Autodesk Inventor part; units mm, degrees
ref_plane "YZ Plane" through (0, 0, 0) normal (1, 0, 0) x (0, 1, 0)
ref_plane "XZ Plane" through (0, 0, 0) normal (0, 1, 0) x (-1, 0, 0)
ref_plane "XY Plane" through (0, 0, 0) normal (0, 0, 1) x (1, 0, 0)
sketch "Sketch1" plane through (0, 0, 0) normal (0, 1, 0) x (-1, 0, 0)
  line L0 (20.193, 15.748) -> (-20.193, 15.748)
  line L1 (-20.193, -15.748) -> (20.193, -15.748)
  line L2 (20.193, 15.748) -> (-20.193, -15.748) construction
  line L3 (-20.193, 15.748) -> (20.193, -15.748) construction
  line L4 (26.2784, 0) -> (13.1572, 0) construction
  line L5 (26.2784, 4.445) -> (20.193, 4.445)
  line L6 (20.193, -4.445) -> (26.2784, -4.445)
  arc A0 (26.2784, -4.445) -> (26.2784, 4.445) centre (26.2784, 0) ccw
  line L7 (0, -15.748) -> (0, 15.748) construction
  line L8 (-26.2784, 4.445) -> (-20.193, 4.445)
  line L9 (-20.193, -4.445) -> (-26.2784, -4.445)
  arc A1 (-26.2784, 4.445) -> (-26.2784, -4.445) centre (-26.2784, 0) ccw
  line L10 (20.193, -15.748) -> (20.193, -4.445)
  line L11 (20.193, 4.445) -> (20.193, 15.748)
  line L12 (-20.193, 15.748) -> (-20.193, 4.445)
  line L13 (-20.193, -4.445) -> (-20.193, -15.748)
  circle A2 centre (-26.2784, 0) radius 2.5527
  circle A3 centre (26.2784, 0) radius 2.5527
  point P0 (0, 0)
  point P1 (19.7178, 0)
  dimension "d0" = 40.386
  dimension "d1" = 31.496
  dimension "d2" = 8.89
  dimension "d5" = 5.1054
  dimension "d6" = 5.1054
extrude "Extrusion2" add sketch "Sketch1" along normal blind 6.35
sketch "Sketch2" plane through (0, 6.35, 0) normal (0, 1, 0) x (1, 0, 0)
  line L0 (20.193, 15.748) -> (-20.193, 15.748)
  line L1 (-20.193, 15.748) -> (20.193, 15.748)
  line L2 (20.193, 15.748) -> (20.193, -15.748)
  line L3 (20.193, -15.748) -> (-20.193, -15.748)
  line L4 (-20.193, -15.748) -> (-20.193, 15.748)
  line L5 (-16.891, -12.446) -> (16.891, -12.446)
  line L6 (16.891, -12.446) -> (16.891, 12.446)
  line L7 (16.891, 12.446) -> (-16.891, 12.446)
  line L8 (-16.891, 12.446) -> (-16.891, -12.446)
  line L9 (-16.891, -12.446) -> (16.891, 12.446) construction
  line L10 (16.891, -12.446) -> (-16.891, 12.446) construction
  point P0 (0, 0)
  dimension "d9" = 3.302
  dimension "d10" = 3.302
extrude "Extrusion3" add sketch "Sketch2" along normal blind 19.05
sketch "Sketch3" plane through (0, 6.35, 0) normal (0, 1, 0) x (1, 0, 0)
  line L0 (-16.891, 12.446) -> (-16.891, -12.446)
  line L1 (-16.891, -12.446) -> (16.891, -12.446)
  line L2 (16.891, 12.446) -> (-16.891, 12.446)
  line L3 (-16.891, 12.446) -> (16.891, 12.446)
  line L4 (16.891, 12.446) -> (16.891, -12.446)
  line L5 (16.891, -12.446) -> (-16.891, -12.446)
  line L6 (-16.891, -12.446) -> (-16.891, 12.446)
  line L7 (-15.875, -11.43) -> (15.875, -11.43)
  line L8 (15.875, -11.43) -> (15.875, 11.43)
  line L9 (15.875, 11.43) -> (-15.875, 11.43)
  line L10 (-15.875, 11.43) -> (-15.875, -11.43)
  line L11 (-15.875, -11.43) -> (15.875, 11.43) construction
  line L12 (15.875, -11.43) -> (-15.875, 11.43) construction
  point P0 (0, 0)
  dimension "d13" = 1.016
  dimension "d14" = 1.016
extrude "Extrusion4" add sketch "Sketch3" along normal blind 5.334
equation "\"d0\" = 2 * imuBoxWallThickness + imuBoardLength + 2 * imuPrintError"
equation "\"d1\" = 2 * imuBoxWallThickness + imuBoardWidth + 2 * imuPrintError"
equation "\"d2\" = widthSlot"
equation "\"d7\" = imuBoxBottom"
equation "\"d9\" = imuBoxWallThickness - imuPrintError"
equation "\"d10\" = imuBoxWallThickness - imuPrintError"
equation "\"d11\" = imuBoxHeight"
equation "\"d15\" = imuBoardBottomThickness"
equation "\"imuBoardWidth\" = 22.86"
equation "\"imuBoardLength\" = 31.75"
equation "\"imuBoardTopThickness\" = 11.176"
equation "\"imuBoardBottomThickness\" = 5.334"
equation "\"imuBoardHoleDistance\" = 19.7104"
equation "\"imuBoxWallThickness\" = 3.81"
equation "\"widthSlot\" = 8.89"
equation "\"imuBoxBottom\" = 6.35"
equation "\"imuBoxHeight\" = 19.05"
equation "\"imuPrintError\" = 0.508"
properties part number "imuBox"
CAD build for the part. Positions are in the model's coordinates, mm. A direction names the side the tool comes from. Round coordinates to 2 decimals unless told otherwise and drop trailing zeros. Order: outer loops, then holes, each group sorted by start corner. A loop starts at its lowest first (then second) coordinate and runs counter-clockwise, first axis right, second up. Notation, with made-up numbers: (24.5, 49) -> (52.5, 49) arc R20 cw to (52.5, 79) -> close; hole circle Ø7 at (44.25, 20.5). An arc over 180 degrees is marked (long way). One line per question, with ' | ' between items.
Q1. Probe probe 1 along Z at (x, y) = (-13, 7); probe 2 along X at (y, z) = (11.5, -6) (3 decimals); probe 3 along X at (y, z) = (22, 5). List the from-to ranges inside material, lowest first.
Completed:
probe 1: z = -15.75 to -11.43, 11.43 to 15.75 | probe 2: x = -20.193 to -15.875, 15.875 to 20.193 | probe 3: x = -20.19 to -16.89, 16.89 to 20.19
Q2. Slice it at B-B (y = 14.5). Write the cut outline in (x, z).
Completed:
outline: (-20.19, -15.75) -> (20.19, -15.75) -> (20.19, 15.75) -> (-20.19, 15.75) -> close; hole (-16.89, -12.45) -> (16.89, -12.45) -> (16.89, 12.45) -> (-16.89, 12.45) -> close
Q3. Drop flat-ended pins along their axis: pin 1 (1.6 mm diameter, centred on y = 9, z = -4, fed in from -X); pin 2 (1 mm diameter, centred on x = -22, y = 11.5, fed in from +Z); pin 3 (2.5 mm diameter, centred on x = 28, z = 0.5, fed in from +Y); pin 4 (2 mm diameter, centred on y = 3, z = 12, fed in from +X). Give the stop position or say it passes through.
Completed:
pin 1: stops at x = -20.19 | pin 2: passes through | pin 3: stops at y = 6.35 | pin 4: stops at x = 20.19
Q4. Which spindle directions (+Z, -Z, +X, -X, +Y, -Y) get a long thin tool onto all of the face, cutting with end or side? Do faces 4 (the flat face through (-23, 3, 4.445)), 5 (the cylindrical face through (-23.73, 3.13, -0.11)), 6 (the flat face through (23, 3, 4.445)), 7 (the flat face through (23, 3, -4.445)), 8 (the flat face through (15.875, 9, 0)). Say none if no direction does.
Completed:
face 4: +Z, -X, +Y, -Y | face 5: +Y, -Y | face 6: +Z, +X, +Y, -Y | face 7: -Z, +X, +Y, -Y | face 8: +Y
Q5. Two-plate mould, pull along X, no slides. Class faces 1 (the cylindrical face through (-30.722, 3.131, 0.098)), 2 (the flat face through (-23, 3, -4.445)), 3 (the flat face through (0, 18, -12.446)): released by +X, released by -X, zero draft, split by the parting line, or undercut.
Completed:
face 1: released by -X | face 2: zero draft | face 3: undercut
Q6. Slice it at A-A (z = 0). Write the cut outline in (x, y) (3 decimals), then the cut area to 3 significant figures.
Completed:
outline: (-30.723, 0) -> (-28.831, 0) -> (-28.831, 6.35) -> (-30.723, 6.35) -> close; (-23.726, 0) -> (23.726, 0) -> (23.726, 6.35) -> (20.193, 6.35) -> (20.193, 25.4) -> (16.891, 25.4) -> (16.891, 11.684) -> (15.875, 11.684) -> (15.875, 6.35) -> (-15.875, 6.35) -> (-15.875, 11.684) -> (-16.891, 11.684) -> (-16.891, 25.4) -> (-20.193, 25.4) -> (-20.193, 6.35) -> (-23.726, 6.35) -> close; (28.831, 0) -> (30.723, 0) -> (30.723, 6.35) -> (28.831, 6.35) -> close | area: 462 mm^2
Q7. Slice it at C-C (z = -6.5). Write the cut outline in (x, y) (3 decimals).
Completed:
outline: (-20.193, 0) -> (20.193, 0) -> (20.193, 25.4) -> (16.891, 25.4) -> (16.891, 11.684) -> (15.875, 11.684) -> (15.875, 6.35) -> (-15.875, 6.35) -> (-15.875, 11.684) -> (-16.891, 11.684) -> (-16.891, 25.4) -> (-20.193, 25.4) -> close
Q8. Slice it at D-D (y = 4.5). Write the cut outline in (x, z) (3 decimals).
Completed:
outline: (-26.278, -4.445) -> (-20.193, -4.445) -> (-20.193, -15.748) -> (20.193, -15.748) -> (20.193, -4.445) -> (26.278, -4.445) arc R4.445 ccw to (26.278, 4.445) -> (20.193, 4.445) -> (20.193, 15.748) -> (-20.193, 15.748) -> (-20.193, 4.445) -> (-26.278, 4.445) arc R4.445 ccw to start; hole circle Ø5.105 at (-26.278, 0); hole circle Ø5.105 at (26.278, 0)
